The listing builds one solid part. Answer for the finished solid, in the listing's coordinates (mm). A direction names the side the tool comes from. Round coordinates to 2 decimals unless told otherwise and drop trailing zeros. Loops run counter-clockwise (first coordinate to the right, second up) from the corner with the lowest first, then second, coordinate; pieces in that order, holes last. Notation, with made-up numbers: M 51,8.5 L 62,8.5 A15 ccw 62,19.5 Z; hole C 33,-1.5 d5. An arc over 180 degrees is marked long. Answer as a JSON object with one key per item and string values.
```python
from build123d import *

# Parameters (mm, degrees)
SKETCH1_R           = 25
SKETCH1_R_2         = 6.5
SKETCH1_W           = 24
SKETCH1_H           = 17.5
SKETCH1_R_3         = 3.249999996
SKETCH1_R_4         = 3.25
BOSS_EXTRUDE1_DEPTH = 26
SKETCH1_3_R         = 10
BOSS_EXTRUDE2_DEPTH = 6
SKETCH1_4_W         = 24
SKETCH1_4_H         = 17.5
BOSS_EXTRUDE3_DEPTH = 19
SKETCH1_5_R         = 10
SKETCH1_5_R_2       = 5
BOSS_EXTRUDE4_DEPTH = 26


with BuildPart() as part:
    # Sketch1 → Boss-Extrude1 (new body)
    # profile 1 of 2: a face of its own
    with BuildSketch(Plane(origin=(0, 0, 0), x_dir=(1, 0, 0), z_dir=(0, 1, 0))):
        with Locations((-70, -38.5)):
            Circle(SKETCH1_R)
        with Locations(Location((-70, -38.5, 0), (0, 0, 90))):
            Circle(SKETCH1_R_2, mode=Mode.SUBTRACT)
    # profile 2 of 2: a face of its own
    with BuildSketch(Plane(origin=(0, 0, 0), x_dir=(1, 0, 0), z_dir=(0, 1, 0))):
        with BuildLine():
            ThreePointArc((-52.650648427, -56.5), (-60.645856533, -61.684046239), (-70, -63.5))
            Line((-70, -63.5), (70, -63.5))
            Line((70, -63.5), (70, 34.217283386))
            ThreePointArc((70, 34.217283386), (60.700640303, 56.667923689), (38.25, 65.967283386))
            ThreePointArc((38.25, 65.967283386), (-37.738740481, 34.900395081), (-92.028760258, -26.679098109))
            ThreePointArc((-92.028760258, -26.679098109), (-85.476895797, -18.866719671), (-76.350661821, -14.320068353))
            ThreePointArc((-76.350661821, -14.320068353), (-26.940104532, 33.755265523), (37.320914143, 58.718486024))
            ThreePointArc((37.320914143, 58.718486024), (59.232009713, 46.90299975), (59.514375282, 22.010790233))
            ThreePointArc((59.514375282, 22.010790233), (57.683425726, 20.172988974), (55.178036419, 19.5))
            Line((55.178036419, 19.5), (51.5, 19.5))
            ThreePointArc((51.5, 19.5), (47.964466094, 18.035533906), (46.5, 14.5))
            Line((46.5, 14.5), (46.5, 11.5))
            ThreePointArc((46.5, 11.5), (47.964466094, 7.964466094), (51.5, 6.5))
            Line((51.5, 6.5), (58, 6.5))
            ThreePointArc((58, 6.5), (61.535533906, 5.035533906), (63, 1.5))
            Line((63, 1.5), (63, -13.5))
            ThreePointArc((63, -13.5), (61.535533906, -17.035533906), (58, -18.5))
            Line((58, -18.5), (51.5, -18.5))
            ThreePointArc((51.5, -18.5), (47.964466094, -19.964466094), (46.5, -23.5))
            Line((46.5, -23.5), (46.5, -26.5))
            ThreePointArc((46.5, -26.5), (45.035533906, -30.035533906), (41.5, -31.5))
            Line((41.5, -31.5), (30, -31.5))
            ThreePointArc((30, -31.5), (26.464466094, -32.964466094), (25, -36.5))
            Line((25, -36.5), (25, -51.5))
            ThreePointArc((25, -51.5), (23.535533906, -55.035533906), (20, -56.5))
            Line((20, -56.5), (-52.650648427, -56.5))
        make_face()
        with Locations((51, -47.75)):
            Rectangle(SKETCH1_W, SKETCH1_H, mode=Mode.SUBTRACT)
        with Locations(Location((51, -25, 0), (0, 0, 90))):
            Circle(SKETCH1_R_3, mode=Mode.SUBTRACT)
        with Locations(Location((63.5, -25, 0), (0, 0, 90))):
            Circle(SKETCH1_R_4, mode=Mode.SUBTRACT)
        with Locations(Location((51, 13, 0), (0, 0, 90))):
            Circle(SKETCH1_R_3, mode=Mode.SUBTRACT)
        with Locations(Location((63.5, 13, 0), (0, 0, 90))):
            Circle(SKETCH1_R_4, mode=Mode.SUBTRACT)
    extrude(amount=BOSS_EXTRUDE1_DEPTH)

    # Sketch1_3 → Boss-Extrude2 (add)
    with BuildSketch(Plane(origin=(0, 0, 0), x_dir=(1, 0, 0), z_dir=(0, 1, 0))):
        with BuildLine():
            ThreePointArc((-45, -38.5), (-46.992025412, -48.279218033), (-52.650648427, -56.5))
            Line((-52.650648427, -56.5), (20, -56.5))
            ThreePointArc((20, -56.5), (23.535533906, -55.035533906), (25, -51.5))
            Line((25, -51.5), (25, -36.5))
            ThreePointArc((25, -36.5), (26.464466094, -32.964466094), (30, -31.5))
            Line((30, -31.5), (41.5, -31.5))
            ThreePointArc((41.5, -31.5), (45.035533906, -30.035533906), (46.5, -26.5))
            Line((46.5, -26.5), (46.5, -23.5))
            ThreePointArc((46.5, -23.5), (47.964466094, -19.964466094), (51.5, -18.5))
            Line((51.5, -18.5), (58, -18.5))
            ThreePointArc((58, -18.5), (61.535533906, -17.035533906), (63, -13.5))
            Line((63, -13.5), (63, 1.5))
            ThreePointArc((63, 1.5), (61.535533906, 5.035533906), (58, 6.5))
            Line((58, 6.5), (51.5, 6.5))
            ThreePointArc((51.5, 6.5), (47.964466094, 7.964466094), (46.5, 11.5))
            Line((46.5, 11.5), (46.5, 14.5))
            ThreePointArc((46.5, 14.5), (47.964466094, 18.035533906), (51.5, 19.5))
            Line((51.5, 19.5), (55.178036419, 19.5))
            ThreePointArc((55.178036419, 19.5), (57.683425726, 20.172988974), (59.514375282, 22.010790233))
            ThreePointArc((59.514375282, 22.010790233), (59.232009713, 46.90299975), (37.320914143, 58.718486024))
            ThreePointArc((37.320914143, 58.718486024), (-26.940104532, 33.755265523), (-76.350661821, -14.320068353))
            ThreePointArc((-76.350661821, -14.320068353), (-54.731839428, -18.703958154), (-45, -38.5))
        make_face()
        with Locations(Location((0, 0, 0), (0, 0, 270))):
            Circle(SKETCH1_3_R, mode=Mode.SUBTRACT)
    extrude(amount=BOSS_EXTRUDE2_DEPTH)

    # Sketch1_4 → Boss-Extrude3 (add)
    with BuildSketch(Plane(origin=(0, 0, 0), x_dir=(1, 0, 0), z_dir=(0, 1, 0))):
        with Locations((51, -47.75)):
            Rectangle(SKETCH1_4_W, SKETCH1_4_H)
    extrude(amount=BOSS_EXTRUDE3_DEPTH)

    # Sketch1_5 → Boss-Extrude4 (add)
    with BuildSketch(Plane(origin=(0, 0, 0), x_dir=(1, 0, 0), z_dir=(0, 1, 0))):
        with Locations(Location((0, 0, 0), (0, 0, 90))):
            Circle(SKETCH1_5_R)
        with Locations(Location((0, 0, 0), (0, 0, 90))):
            Circle(SKETCH1_5_R_2, mode=Mode.SUBTRACT)
    extrude(amount=BOSS_EXTRUDE4_DEPTH)


solid = part.part
```
Item 1: The part is cut by section C-C (x = 0). Give the vertices of the cut face in (y, z), then the cut area to 3 significant figures.
Values follow:
{"outline": "M 0,-55.44 L 26,-55.44 L 26,-47.89 L 6,-47.89 L 6,-10 L 26,-10 L 26,-5 L 0,-5 Z; M 0,5 L 26,5 L 26,10 L 6,10 L 6,56.5 L 26,56.5 L 26,63.5 L 0,63.5 Z", "area": "1,140 mm^2"}
Item 2: The part is cut by section D-D (z = -44). Give the vertices of the cut face in (x, y), then the cut area to 3 significant figures.
Values follow:
{"outline": "M -23.59,0 L 68.46,0 L 68.46,26 L 60.73,26 L 60.73,6 L -8.65,6 L -8.65,26 L -23.59,26 Z", "area": "1,010 mm^2"}
Item 3: Which of the six approach directions +Z, -Z, +X, -X, +Y, -Y give full straight-line access (tool end or side, diameter ignored) to faces 1 (the face through (60.278, 12.818, -12.577)), 2 (the face through (55, 16, 18.5))?
Values follow:
{"face 1": "+Y, -Y", "face 2": "+Y"}
Item 4: Flat-ended cylindrical pins translate along their axes: P1, Ø5, axis at x = 55, y = 11.5, coming from the -Z side; P2, Ø3.5, axis at y = 13.5, z = -13, coming from the -X side; P3, Ø7.5, axis at y = 16.5, z = 42, coming from the -X side. Find the tip coordinate at first contact, or state that the pin passes through.
Values follow:
{"P1": "z = -62.59", "P2": "x = -64.8", "P3": "x = -95"}
Item 5: Determine the mould class of faces 3 (the face through (61.5, 15.86, -5.07)), 4 (the face through (-36.79, 12.82, -35.57)), 5 (the face through (51, 22, 39)), 6 (the face through (-50, 26, 27)) for opening direction X: released by +X, released by -X, zero draft, split by the parting line, or undercut.
Values follow:
{"face 3": "undercut", "face 4": "released by -X", "face 5": "undercut", "face 6": "zero draft"}
Item 6: Straight lines are drawn through the part: line 1 (X direction, y = 16, z = 38.5); line 2 (Z direction, x = 51, y = 11.5); line 3 (X direction, y = 21.5, z = -11.5). For each, find the intervals that lie inside material, in ascending order.
Values follow:
{"line 1": "-95 to -76.5, -63.5 to -45, 25 to 70", "line 2": "-63.29 to -55.16, -19.47 to -16.25, -9.75 to -6.53, 18.53 to 21.75, 28.25 to 63.5", "line 3": "-64.57 to -54.78, 46.5 to 48.12, 53.88 to 60.62, 66.38 to 70"}
Item 7: The part is cut by section A-A (y = 8). Give the number of separate pieces and of enclosed holes in the cut face, then the cut area to 3 significant figures.
Values follow:
{"separate pieces": "2", "enclosed holes": "7", "area": "6,240 mm^2"}
